from build123d import *

# Parameters (mm, degrees)
BOSS_EXTRUDE1_DEPTH  = 3.175
M4_CLEARANCE_HOLE1_D = 4.5


with BuildPart() as part:
    # Sketch1 → Boss-Extrude1 (new body)
    with BuildSketch(Plane.XY):
        with BuildLine():
            Line((37.350187889, -76.716042997), (65.516187889, -76.716042997))
            Line((65.516187889, -76.716042997), (65.516187889, -80.125742997))
            ThreePointArc((65.516187889, -80.125742997), (71.016187889, -85.625742997), (76.516187889, -80.125742997))
            Line((76.516187889, -80.125742997), (76.516187889, -76.716042997))
            Line((76.516187889, -76.716042997), (104.682187889, -76.716042997))
            ThreePointArc((104.682187889, -76.716042997), (106.256649797, -76.606152124), (107.800580738, -76.278610439))
            Line((107.800580738, -76.278610439), (111.218470842, -79.696500543))
            ThreePointArc((111.218470842, -79.696500543), (118.996645435, -79.696500543), (118.996645435, -71.91832595))
            Line((118.996645435, -71.91832595), (115.578755331, -68.500435846))
            ThreePointArc((115.578755331, -68.500435846), (115.906297016, -66.956504905), (116.016187889, -65.382042997))
            Line((116.016187889, -65.382042997), (116.016187889, -33.716042997))
            Line((116.016187889, -33.716042997), (119.425887889, -33.716042997))
            ThreePointArc((119.425887889, -33.716042997), (124.925887889, -28.216042997), (119.425887889, -22.716042997))
            Line((119.425887889, -22.716042997), (116.016187889, -22.716042997))
            Line((116.016187889, -22.716042997), (116.016187889, 8.949957003))
            ThreePointArc((116.016187889, 8.949957003), (115.906297016, 10.524418912), (115.578755331, 12.068349853))
            Line((115.578755331, 12.068349853), (118.996645435, 15.486239957))
            ThreePointArc((118.996645435, 15.486239957), (118.996645435, 23.26441455), (111.218470842, 23.26441455))
            Line((111.218470842, 23.26441455), (107.800580738, 19.846524446))
            ThreePointArc((107.800580738, 19.846524446), (106.256649797, 20.174066131), (104.682187889, 20.283957003))
            Line((104.682187889, 20.283957003), (76.516187889, 20.283957003))
            Line((76.516187889, 20.283957003), (76.516187889, 23.693657003))
            ThreePointArc((76.516187889, 23.693657003), (71.016187889, 29.193657003), (65.516187889, 23.693657003))
            Line((65.516187889, 23.693657003), (65.516187889, 20.283957003))
            Line((65.516187889, 20.283957003), (37.350187889, 20.283957003))
            ThreePointArc((37.350187889, 20.283957003), (35.77572598, 20.174066131), (34.231795039, 19.846524446))
            Line((34.231795039, 19.846524446), (30.813904935, 23.26441455))
            ThreePointArc((30.813904935, 23.26441455), (23.035730342, 23.26441455), (23.035730342, 15.486239957))
            Line((23.035730342, 15.486239957), (26.453620446, 12.068349853))
            ThreePointArc((26.453620446, 12.068349853), (26.126078761, 10.524418912), (26.016187889, 8.949957003))
            Line((26.016187889, 8.949957003), (26.016187889, -22.716042997))
            Line((26.016187889, -22.716042997), (22.606487889, -22.716042997))
            ThreePointArc((22.606487889, -22.716042997), (17.106487889, -28.216042997), (22.606487889, -33.716042997))
            Line((22.606487889, -33.716042997), (26.016187889, -33.716042997))
            Line((26.016187889, -33.716042997), (26.016187889, -65.382042997))
            ThreePointArc((26.016187889, -65.382042997), (26.126078761, -66.956504905), (26.453620446, -68.500435846))
            Line((26.453620446, -68.500435846), (23.035730342, -71.91832595))
            ThreePointArc((23.035730342, -71.91832595), (23.035730342, -79.696500543), (30.813904935, -79.696500543))
            Line((30.813904935, -79.696500543), (34.231795039, -76.278610439))
            ThreePointArc((34.231795039, -76.278610439), (35.77572598, -76.606152124), (37.350187889, -76.716042997))
        make_face()
    extrude(amount=BOSS_EXTRUDE1_DEPTH)

    # M4 Clearance Hole1 (through all)
    with Locations(Plane.XY.offset(3.175)):
        with Locations((26.924817639, -75.807413246), (22.606487889, -28.216042997), (71.016187889, -80.125742997), (115.107558138, -75.807413246), (119.425887889, -28.216042997), (115.107558138, 19.375327253), (71.016187889, 23.693657003), (26.924817639, 19.375327253)):
            Hole(M4_CLEARANCE_HOLE1_D / 2)


solid = part.part
For this review, take the finished solid that the model builds, in its own axes (mm). A direction names the side the tool comes from. Round coordinates to 2 decimals unless told otherwise and drop trailing zeros. Loops run counter-clockwise (first coordinate to the right, second up) from the corner with the lowest first, then second, coordinate; pieces in that order, holes last. Notation, with made-up numbers: (4, 89.25) - (45, 89.25) arc R23 cw to (45, 124.25) - close; hole circle Ø9 at (86.5, 39.5). An arc over 180 degrees is marked (long way). One line per item, written item: value. Start each with the question number.
Item 1: For faces 1 (the flat face through (118, -22.716, 2)), 2 (the cylindrical face through (35.754, -76.603, 1.565)), 3 (the flat face through (52, 20.284, 2)), 4 (the flat face through (26.016, -7, 2)), list the 3-axis set-ups (+Z, -Z, +X, -X, +Y, -Y) from which the entire face can be reached by the end or side of a thin tool; tool diameter is ignored.
Item 2: For L1, parallel to X at y = -77.5, z = 1.9; L2, parallel to Y at x = 115.5, z = 1.85; L3, parallel to Y at x = 23.5, z = 1.5, list the stretches that pass through material, from the lowest coordinate up.
Item 3: Take a section at A-A (y = -17). Give the boundary of the cut face in (x, z) (3 decimals).
Item 4: Take a section at B-B (x = 92). Give the boundary of the cut face in (y, z) (3 decimals).
Item 5: The part is to be moulded in two halves that separate along Y. For faces 5 (the cylindrical face through (115.9, -67, 1.6)), 6 (the flat face through (70, -27, 0)), 7 (the cylindrical face through (26.123, -66.935, 1.565)), 8 (the flat face through (109.533, 21.579, 1.565)), say which applies: +Y half, -Y half, draft (parallel to the pull), parting line (faces both ways), or undercut.
Item 6: Take a section at C-C (z = 1.65). State how many separate pieces and enclosed holes the cut face has, plus the area to 3 significant figures.
Item 7: Clearance check with flat-ended pins moving along their axes: pin 1 Ø1.6 at (x, z) = (56, 1) entering from -Y; pin 2 Ø1.6 at (y, z) = (-79, 2) entering from +X; pin 3 Ø7 at (x, y) = (115.11, 19.38) entering from -Z; pin 4 Ø1 at (y, z) = (22, 2) entering from -X. State where each tip first meets the part, or that it passes through.
Answer below:
1. face 1: +Z, -Z, +X
1. face 2: +Z, -Z, -Y
1. face 3: +Z, -Z, +Y
1. face 4: +Z, -Z, -X
2. L1: x = 21.69 to 25.44, 28.41 to 33.01, 65.52 to 76.52, 109.02 to 113.63, 116.59 to 120.34
2. L2: y = -81.29 to -78.02, -73.59 to 17.16, 21.59 to 24.86
2. L3: y = -80.11 to -71.45, -33.72 to -30.28, -26.15 to -22.72, 15.02 to 23.68
3. outline: (26.016, 0) - (116.016, 0) - (116.016, 3.175) - (26.016, 3.175) - close
4. outline: (-76.716, 0) - (20.284, 0) - (20.284, 3.175) - (-76.716, 3.175) - close
5. face 5: undercut
5. face 6: draft
5. face 7: undercut
5. face 8: +Y half
6. separate pieces: 1
6. enclosed holes: 8
6. area: 9,190 mm2
7. pin 1: stops at y = -76.72
7. pin 2: stops at x = 120.06
7. pin 3: stops at z = 0
7. pin 4: stops at x = 21.85
